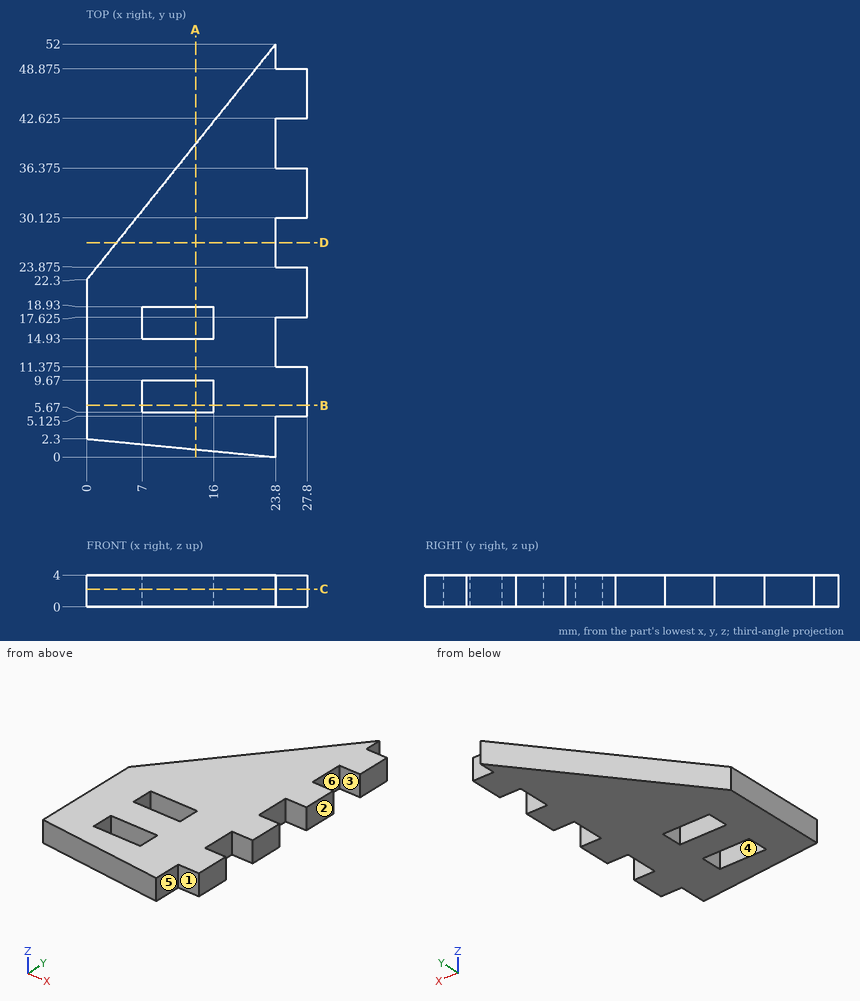
Here's the drawing with two shaded views (mm, measured from the low corner). I have some questions. A direction names the side the tool comes from. Give positions to 0.01 mm unless a question says otherwise; leave off trailing zeros. Order: outer loops, then holes, each group sorted by start corner. A loop starts at its lowest first (then second) coordinate and runs counter-clockwise, first axis right, second up. Notation, with made-up numbers: (13.25, 36.25) -> (39.25, 36.25) arc R12 cw to (39.25, 50.25) -> close; hole circle Ø10 at (22.5, 32). An arc over 180 degrees is marked (long way). Use a Markdown table: item, result. Add a question column.
Item 1: For the marked faces 4, 5 and 6, which set-ups out of +Z, -Z, +X, -X, +Y, -Y let a thin tool reach every point of the face, with its end or its side?
Item 2: Will these pins go through, and if not, where does the flat tip stop? pin 1 (1.2 mm diameter, centred on x = 9.5, z = 1, fed in from -Y); pin 2 (2 mm diameter, centred on x = 11, z = 2, fed in from +Y); pin 3 (1.2 mm diameter, centred on x = 12.5, z = 1.5, fed in from -Y).
Item 3: Imagine slicing it at D-D on y = 27. Please give me the cut outline in (x, z).
Item 4: Imagine slicing it at A-A on x = 13.75. Please give me the cut outline in (y, z), plus the area to 3 significant figures.
Item 5: Imagine slicing it at C-C on z = 2.25. Please give me the cut outline in (x, y) (3 decimals).
Item 6: Imagine slicing it at B-B on y = 6.5. Please give me the cut outline in (x, z).
Item 7: I need wall thicknesses on line 1 (Y direction, x = 26.5, z = 3.55) (3 decimals); line 2 (X direction, y = 8, z = 2.3); line 3 (Y direction, x = 15.75, z = 1.2). Which ranges of each line are inside material? Lowest first, please.
Item 8: If we mould it in two halves opening along Y, with no side actions, what happens to the marked faces 1, 2 and 3? For each: pulls with the +Y half, pulls with the -Y half, needs draft (parallel to the pull), parting line crosses it, or undercut.
Data:
| question | item | result |
|---|---|---|
| 1 | face 4 | +Z, -Z |
| 1 | face 5 | +Z, -Z, +X, -Y |
| 1 | face 6 | +Z, -Z, +X |
| 2 | pin 1 | stops at y = 1.32 |
| 2 | pin 2 | stops at y = 37.27 |
| 2 | pin 3 | stops at y = 1.03 |
| 3 | outline | (3.77, 0) -> (23.8, 0) -> (23.8, 4) -> (3.77, 4) -> close |
| 4 | outline | (0.97, 0) -> (5.67, 0) -> (5.67, 4) -> (0.97, 4) -> close; (9.67, 0) -> (14.93, 0) -> (14.93, 4) -> (9.67, 4) -> close; (18.93, 0) -> (39.46, 0) -> (39.46, 4) -> (18.93, 4) -> close |
| 4 | area | 122 mm² |
| 5 | outline | (0, 2.3) -> (23.8, 0) -> (23.8, 5.125) -> (27.8, 5.125) -> (27.8, 11.375) -> (23.8, 11.375) -> (23.8, 17.625) -> (27.8, 17.625) -> (27.8, 23.875) -> (23.8, 23.875) -> (23.8, 30.125) -> (27.8, 30.125) -> (27.8, 36.375) -> (23.8, 36.375) -> (23.8, 42.625) -> (27.8, 42.625) -> (27.8, 48.875) -> (23.8, 48.875) -> (23.8, 52) -> (0, 22.3) -> close; hole (7, 5.67) -> (16, 5.67) -> (16, 9.67) -> (7, 9.67) -> close; hole (7, 14.93) -> (16, 14.93) -> (16, 18.93) -> (7, 18.93) -> close |
| 6 | outline | (0, 0) -> (7, 0) -> (7, 4) -> (0, 4) -> close; (16, 0) -> (27.8, 0) -> (27.8, 4) -> (16, 4) -> close |
| 7 | line 1 | y = 5.125 to 11.375, 17.625 to 23.875, 30.125 to 36.375, 42.625 to 48.875 |
| 7 | line 2 | x = 0 to 7, 16 to 27.8 |
| 7 | line 3 | y = 0.78 to 5.67, 9.67 to 14.93, 18.93 to 41.95 |
| 8 | face 1 | pulls with the -Y half |
| 8 | face 2 | needs draft |
| 8 | face 3 | undercut |
